Geometry check sheet. Reference: the model listing, model coordinates, mm. A direction names the side the tool comes from. Round coordinates to 2 decimals unless told otherwise and drop trailing zeros. Order: outer loops, then holes, each group sorted by start corner. A loop starts at its lowest first (then second) coordinate and runs counter-clockwise, first axis right, second up. Notation, with made-up numbers: (17.25, -16.75) - (44.25, -16.75) arc R29 ccw to (44.25, 12.25) - close; hole circle Ø10 at (-38.75, 37). An arc over 180 degrees is marked (long way). Use a Markdown table: item, result. Add a question column.
(1) Section check A-A on y = 38. Give the number of separate pieces and of enclosed holes in the cut face, then the cut area to 3 significant figures.
(2) Mould release check, pull along Z, two halves, no side actions. Record for faces 1 (the face through (20, 76.2, 1)), 2 (the face through (-20, 38.63, -46.12)): released by +Z, released by -Z, zero draft, split by the parting line, or undercut.
(3) Thickness scan on line 1 along Z through (x, y) = (40, 3); line 2 along Z through (x, y) = (-74.5, 39.5); line 3 along X through (y, z) = (62, -46). Record the ranges inside material, lowest first. Write a range as [from, to].
(4) Gauge pin test, flat ends, axial feed: P1, Ø5, axis at x = -49, y = 53, coming from the +Z side; P2, Ø2, axis at x = 59.5, z = 7, coming from the +Y side; P3, Ø1, axis at x = -30.5, y = 75, coming from the -Z side; P4, Ø3, axis at x = 3, z = 19.5, coming from the +Y side. Record the tip position at first contact, or that the pin passes through.
(5) Access from +Z, -Z, +X, -X, +Y, -Y to the whole of each face (thin tool, end or side, straight path). Record for faces 3 (the face through (-87.2, 38.6, 17.3)), 4 (the face through (0, -25.4, 0)).
(6) Section check D-D on y = 87.5. Record the boundary of the cut face in (x, z).
```python
from build123d import *

# Parameters (mm, degrees)
SKETCH2_R           = 101.6
BOSS_EXTRUDE1_DEPTH = 76.2
SKETCH4_R           = 12.7
BOSS_EXTRUDE4_DEPTH = 25.4
FILLET1_R           = 5.08
FILLET2_R           = 5.08
CUT_EXTRUDE2_START  = -76.2
CUT_EXTRUDE2_DEPTH  = 76.2
BOSS_EXTRUDE5_START = 25.4
SKETCH8_R           = 12.7
BOSS_EXTRUDE5_DEPTH = 25.4


# Read off the part's stored shape, not the designer's step: Cut-Extrude2
with BuildPart() as part:
    # Sketch2 → Boss-Extrude1 (new body)
    with BuildSketch(Plane(origin=(0, 0, 0), x_dir=(1, 0, 0), z_dir=(0, 1, 0))):
        with Locations(Location((0, 0, 0), (0, 0, 90))):
            Circle(SKETCH2_R)
    extrude(amount=BOSS_EXTRUDE1_DEPTH)

    # Sketch4 → Boss-Extrude4 (add)
    with BuildSketch(Plane(origin=(0, 0, 0), x_dir=(-1, 0, 0), z_dir=(0, -1, 0))):
        with Locations(Location((0, 0, 0), (0, 0, 270))):
            Circle(SKETCH4_R)
    extrude(amount=BOSS_EXTRUDE4_DEPTH)

    # Fillet1
    fillet1_edges = [part.edges().sort_by_distance(p)[0] for p in [
        (0, 76.2, 101.6),
    ]]
    fillet(fillet1_edges, radius=FILLET1_R)

    # Fillet2
    fillet2_edges = [part.edges().sort_by_distance(p)[0] for p in [
        (0, 0, 101.6),
    ]]
    fillet(fillet2_edges, radius=FILLET2_R)

    # Cut-Extrude2 outline → Cut-Extrude2 (cut)
    with BuildSketch(Plane.XZ.offset(CUT_EXTRUDE2_START)):
        with BuildLine():
            ThreePointArc((12.696427962, 0.301192634), (12.464886183, -2.432408777), (11.651702143, -5.052508009))
            Line((11.651702143, -5.052508009), (81.561914999, -35.367556061))
            ThreePointArc((81.561914999, -35.367556061), (87.254203278, -17.026861436), (88.874995735, 2.108348439))
            Line((88.874995735, 2.108348439), (12.696427962, 0.301192634))
        make_face()
        with BuildLine():
            ThreePointArc((8.764754955, 9.190705663), (10.533978287, 7.094032806), (11.811660273, 4.666334922))
            Line((11.811660273, 4.666334922), (82.681621907, 32.664344457))
            ThreePointArc((82.681621907, 32.664344457), (73.737848009, 49.658229641), (61.353284684, 64.33493964))
            Line((61.353284684, 64.33493964), (8.764754955, 9.190705663))
        make_face()
        with BuildLine():
            Line((64.33493964, -61.353284684), (9.190705663, -8.764754955))
            ThreePointArc((9.190705663, -8.764754955), (7.094032806, -10.533978287), (4.666334922, -11.811660273))
            Line((4.666334922, -11.811660273), (32.664344457, -82.681621907))
            ThreePointArc((32.664344457, -82.681621907), (49.658229641, -73.737848009), (64.33493964, -61.353284684))
        make_face()
        with BuildLine():
            ThreePointArc((-0.301192634, 12.696427962), (2.432408777, 12.464886183), (5.052508009, 11.651702143))
            Line((5.052508009, 11.651702143), (35.367556061, 81.561914999))
            ThreePointArc((35.367556061, 81.561914999), (17.026861436, 87.254203278), (-2.108348439, 88.874995735))
            Line((-2.108348439, 88.874995735), (-0.301192634, 12.696427962))
        make_face()
        with BuildLine():
            Line((2.108348439, -88.874995735), (0.301192634, -12.696427962))
            ThreePointArc((0.301192634, -12.696427962), (-2.432408777, -12.464886183), (-5.052508009, -11.651702143))
            Line((-5.052508009, -11.651702143), (-35.367556061, -81.561914999))
            ThreePointArc((-35.367556061, -81.561914999), (-17.026861436, -87.254203278), (2.108348439, -88.874995735))
        make_face()
        with BuildLine():
            ThreePointArc((-9.190705663, 8.764754955), (-7.094032806, 10.533978287), (-4.666334922, 11.811660273))
            Line((-4.666334922, 11.811660273), (-32.664344457, 82.681621907))
            ThreePointArc((-32.664344457, 82.681621907), (-49.658229641, 73.737848009), (-64.33493964, 61.353284684))
            Line((-64.33493964, 61.353284684), (-9.190705663, 8.764754955))
        make_face()
        with BuildLine():
            Line((-61.353284684, -64.33493964), (-8.764754955, -9.190705663))
            ThreePointArc((-8.764754955, -9.190705663), (-10.533978287, -7.094032806), (-11.811660273, -4.666334922))
            Line((-11.811660273, -4.666334922), (-82.681621907, -32.664344457))
            ThreePointArc((-82.681621907, -32.664344457), (-73.737848009, -49.658229641), (-61.353284684, -64.33493964))
        make_face()
        with BuildLine():
            ThreePointArc((-12.696427962, -0.301192634), (-12.464886183, 2.432408777), (-11.651702143, 5.052508009))
            Line((-11.651702143, 5.052508009), (-81.561914999, 35.367556061))
            ThreePointArc((-81.561914999, 35.367556061), (-87.254203278, 17.026861436), (-88.874995735, -2.108348439))
            Line((-88.874995735, -2.108348439), (-12.696427962, -0.301192634))
        make_face()
    extrude(amount=CUT_EXTRUDE2_DEPTH, mode=Mode.SUBTRACT)

    # Sketch8 → Boss-Extrude5 (add)
    with BuildSketch(Plane(origin=(0, 76.2, 0), x_dir=(1, 0, 0), z_dir=(0, 1, 0)).offset(BOSS_EXTRUDE5_START)):
        with Locations(Location((0, 0, 0), (0, 0, 270))):
            Circle(SKETCH8_R)
    extrude(amount=-BOSS_EXTRUDE5_DEPTH)


solid = part.part
```
Check sheet entries:
| question | item | result |
|---|---|---|
| 1 | separate pieces | 1 |
| 1 | enclosed holes | 8 |
| 1 | area | 19,000 mm2 |
| 2 | face 1 | zero draft |
| 2 | face 2 | undercut |
| 3 | line 1 | z = [-92.91, -79.39], [-38.15, -17.35], [0.95, 15.8], [41.94, 92.91] |
| 3 | line 2 | z = [-69.08, -48.51], [-29.43, -1.77], [32.31, 69.08] |
| 3 | line 3 | x = [-90.59, -76.07], [-43.87, -19.95], [1.09, 18.17], [48.24, 90.59] |
| 4 | P1 | stops at z = 90.33 |
| 4 | P2 | stops at y = 76.2 |
| 4 | P3 | stops at z = -95.59 |
| 4 | P4 | passes through |
| 5 | face 3 | +Y, -Y |
| 5 | face 4 | +Z, -Z, +X, -X, -Y |
| 6 | outline | circle Ø25.4 at (0, 0) |
